Build history of the part. All positions in model axes, mm. Face numbers are marked on the shaded views. Give positions to 0.01 mm unless a question says otherwise; leave off trailing zeros. Order: outer loops, then holes, each group sorted by start corner. A loop starts at its lowest first (then second) coordinate and runs counter-clockwise, first axis right, second up. Notation, with made-up numbers: (10.25, -9.5) -> (43.25, -9.5) arc R28 ccw to (43.25, 17.5) -> close; hole circle Ø10 at (20.5, 57.5). An arc over 180 degrees is marked (long way). One line per question, with ' | ' between items. Start each with the question number.
(1) Cut at A-A (x = 0). Give the cut face in (y, z).
(2) Pin check, flat tip, straight feed: pin 1 Ø2.5 at (x, z) = (51.85, -3.23) entering from -Y. Stop position of the tip, or through.
(3) Pull direction Y, two halves, no side cores. Call the marked faces 1 and 2: +Y half, -Y half, draft (parallel to the pull), parting line (faces both ways), or undercut.
(4) Drill centre lines: L1, parallel to Z at x = 50.5, y = -0.05; L2, parallel to Z at x = 0, y = -0.25; L3, parallel to X at y = -0.05, z = 27. Where is each one in solid material? Low to high. Write a range as from..to.
(5) Cut at C-C (y = -0.15). Give the cut face in (x, z), then the cut area to 3 significant figures.
(6) Cut at B-B (z = 0). Give the cut face in (x, y), then the cut area to 3 significant figures.
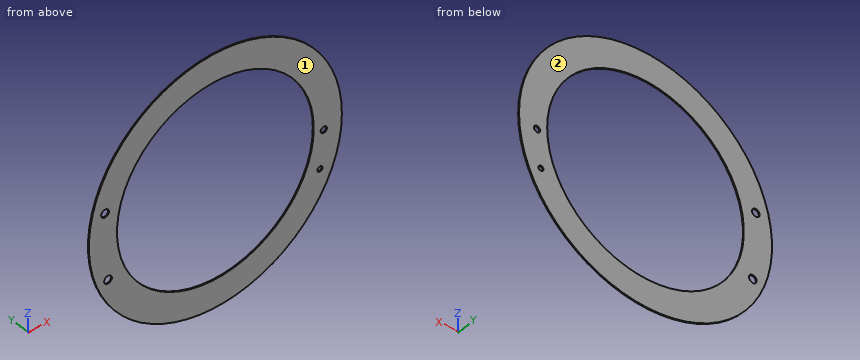
from build123d import *

# Parameters (mm, degrees)
F0_R     = 60.484024
F0_R_2   = 1.857944
F0_R_3   = 1.231078
F0_R_4   = 1.503057
F0_R_5   = 1.860203
F0_R_6   = 47.023522
F1_DEPTH = 0.508


with BuildPart() as f1:
    # F0 (on Front) → F1 (new body)
    with BuildSketch(Plane.XZ):
        Circle(F0_R)
        with Locations((-51.31948, -20.179848)):
            Circle(F0_R_2, mode=Mode.SUBTRACT)
        with Locations((49.991365, -20.913929)):
            Circle(F0_R_3, mode=Mode.SUBTRACT)
        with Locations((51.846373, -3.229027)):
            Circle(F0_R_4, mode=Mode.SUBTRACT)
        with Locations((-52.730181, 12.048138)):
            Circle(F0_R_5, mode=Mode.SUBTRACT)
        Circle(F0_R_6, mode=Mode.SUBTRACT)
    extrude(amount=F1_DEPTH)


solid = f1.part
Result set:
1) outline: (-0.51, -60.48) -> (0, -60.48) -> (0, -47.02) -> (-0.51, -47.02) -> close; (-0.51, 47.02) -> (0, 47.02) -> (0, 60.48) -> (-0.51, 60.48) -> close
2) pin 1: passes through
3) face 1: -Y half | face 2: +Y half
4) L1: z = -33.29..-22.04, -19.79..-3.9, -2.56..33.29 | L2: z = -60.48..-47.02, 47.02..60.48 | L3: x = -54.12..-38.5, 38.5..54.12
5) outline: circle Ø120.97 at (0, 0); hole circle Ø3.72 at (-52.73, 12.05); hole circle Ø3.72 at (-51.32, -20.18); hole circle Ø94.05 at (0, 0); hole circle Ø2.46 at (49.99, -20.91); hole circle Ø3.01 at (51.85, -3.23) | area: 4,510 mm2
6) outline: (-60.48, -0.51) -> (-47.02, -0.51) -> (-47.02, 0) -> (-60.48, 0) -> close; (47.02, -0.51) -> (60.48, -0.51) -> (60.48, 0) -> (47.02, 0) -> close | area: 13.7 mm2
